Can you work these out from the model? Positions are in its coordinate system, mm. A direction names the side the tool comes from. Coordinates: 2 decimals unless noted, no trailing zeros. Write each loop counter-clockwise with the first axis right and the second up, starting at its lowest first coordinate (ties: lowest second). Pieces come first, ordered by that corner, then holes. Notation, with made-up numbers: M 59.25,13.25 L 88.25,13.25 A23 ccw 88.25,46.25 Z; hole C -33,3.25 d10. An arc over 180 degrees is marked long. Use one line per item in the form item = value. Start each with the question number.
```python
from build123d import *

# Parameters (mm, degrees)
SKETCH1_W           = 3
SKETCH1_H           = 7
BOSS_EXTRUDE1_DEPTH = 6
SKETCH5_W           = 70
SKETCH5_H           = 6
CUT_EXTRUDE2_DEPTH  = 2
SKETCH6_R           = 3
CUT_EXTRUDE3_DEPTH  = 10


with BuildPart() as part:
    # Sketch1 → Boss-Extrude1 (new body)
    # profile 1 of 3: a face of its own
    with BuildSketch(Plane.XY):
        with BuildLine():
            ThreePointArc((0.112083698, 404.617647059), (2.612083698, 407.117647059), (5.112083698, 404.617647059))
            Line((5.112083698, 404.617647059), (18.529411765, 404.617647059))
            Line((18.529411765, 404.617647059), (18.529411765, 419.117647059))
            ThreePointArc((18.529411765, 419.117647059), (17.064945671, 422.653180965), (13.529411765, 424.117647059))
            Line((13.529411765, 424.117647059), (-46.470588235, 424.117647059))
            ThreePointArc((-46.470588235, 424.117647059), (-50.006122141, 422.653180965), (-51.470588235, 419.117647059))
            Line((-51.470588235, 419.117647059), (-51.470588235, 404.617647059))
            Line((-51.470588235, 404.617647059), (-42.310598324, 404.617647059))
            ThreePointArc((-42.310598324, 404.617647059), (-39.810598324, 407.117647059), (-37.310598324, 404.617647059))
            Line((-37.310598324, 404.617647059), (0.112083698, 404.617647059))
        make_face()
    # profile 2 of 3: a face of its own
    with BuildSketch(Plane.XY):
        with BuildLine():
            Line((18.529411765, 404.617647059), (5.112083698, 404.617647059))
            ThreePointArc((5.112083698, 404.617647059), (2.612083698, 402.117647059), (0.112083698, 404.617647059))
            Line((0.112083698, 404.617647059), (-37.310598324, 404.617647059))
            ThreePointArc((-37.310598324, 404.617647059), (-39.810598324, 402.117647059), (-42.310598324, 404.617647059))
            Line((-42.310598324, 404.617647059), (-51.470588235, 404.617647059))
            Line((-51.470588235, 404.617647059), (-51.470588235, 373.617647059))
            Line((-51.470588235, 373.617647059), (-42.310598324, 373.617647059))
            ThreePointArc((-42.310598324, 373.617647059), (-39.810598324, 376.117647059), (-37.310598324, 373.617647059))
            Line((-37.310598324, 373.617647059), (0.112083698, 373.617647059))
            ThreePointArc((0.112083698, 373.617647059), (2.612083698, 376.117647059), (5.112083698, 373.617647059))
            Line((5.112083698, 373.617647059), (18.529411765, 373.617647059))
            Line((18.529411765, 373.617647059), (18.529411765, 404.617647059))
        make_face()
        with Locations((-46.970588235, 389.117647059)):
            Rectangle(SKETCH1_W, SKETCH1_H, mode=Mode.SUBTRACT)
        with Locations((14.029411765, 389.117647059)):
            Rectangle(SKETCH1_W, SKETCH1_H, mode=Mode.SUBTRACT)
    # profile 3 of 3: a face of its own
    with BuildSketch(Plane.XY):
        with BuildLine():
            Line((18.529411765, 359.117647059), (18.529411765, 373.617647059))
            Line((18.529411765, 373.617647059), (5.112083698, 373.617647059))
            ThreePointArc((5.112083698, 373.617647059), (2.612083698, 371.117647059), (0.112083698, 373.617647059))
            Line((0.112083698, 373.617647059), (-37.310598324, 373.617647059))
            ThreePointArc((-37.310598324, 373.617647059), (-39.810598324, 371.117647059), (-42.310598324, 373.617647059))
            Line((-42.310598324, 373.617647059), (-51.470588235, 373.617647059))
            Line((-51.470588235, 373.617647059), (-51.470588235, 359.117647059))
            ThreePointArc((-51.470588235, 359.117647059), (-50.006122141, 355.582113153), (-46.470588235, 354.117647059))
            Line((-46.470588235, 354.117647059), (13.529411765, 354.117647059))
            ThreePointArc((13.529411765, 354.117647059), (17.064945671, 355.582113153), (18.529411765, 359.117647059))
        make_face()
    extrude(amount=BOSS_EXTRUDE1_DEPTH)

    # Sketch5 → Cut-Extrude2 (cut)
    with BuildSketch(Plane.XY.offset(6)):
        with Locations((-16.470588235, 389.117647059)):
            Rectangle(SKETCH5_W, SKETCH5_H)
    extrude(amount=-CUT_EXTRUDE2_DEPTH, mode=Mode.SUBTRACT)

    # Sketch6 → Cut-Extrude3 (cut)
    with BuildSketch(Plane.XY.offset(4)):
        with Locations((-16.470588235, 389.117647059)):
            Circle(SKETCH6_R)
    extrude(amount=-CUT_EXTRUDE3_DEPTH, mode=Mode.SUBTRACT)


solid = part.part
```
1) Suppose I cut it at B-B on x = 4. Please give me the cut outline in (y, z).
2) Suppose I cut it at D-D on y = 372.5. Please give me the cut outline in (x, z).
3) Suppose I cut it at A-A on y = 387.5. Please give me the cut outline in (x, z).
4) Please list where these lines run through material, in increasing order: line 1 (Y direction, x = -40, z = 4.75); line 2 (Y direction, x = -26.5, z = 4.95); line 3 (Y direction, x = -39, z = 4.95).
5) Which directions (+Z, -Z, +X, -X, +Y, -Y) give clear straight access to the entire face, cutting with the end or side of a thin tool? Please do faces 1 (the face through (-47, 392.618, 3)), 2 (the face through (17.104, 422.614, 2.958)), 3 (the face through (-17, 386.118, 5)).
6) If we mould it in two halves opening along Y, with no side actions, what happens to faces 4 (the face through (17, 392.118, 5)), 5 (the face through (-2, 389, 4)), 6 (the face through (-17, 370, 6)), 7 (the face through (17.026, 355.543, 2.958))? For each: +Y half, -Y half, draft (parallel to the pull), parting line (faces both ways), or undercut.
7) Will these pins go through, and if not, where does the flat tip stop? pin 1 Ø4 at (x, y) = (2.61, 404.62) entering from -Z; pin 2 Ø5 at (x, y) = (-27, 389.5) entering from +Z; pin 3 Ø1 at (x, z) = (17, 5) entering from -Y; pin 4 Ø1.6 at (x, z) = (16.5, 5) entering from +Y.
8) Suppose I cut it at C-C on z = 2.1. Please give me the cut outline in (x, y), and give its area (3 significant figures).
Computed values:
q1.outline = M 354.12,0 L 371.54,0 L 371.54,6 L 354.12,6 Z; M 375.7,0 L 402.54,0 L 402.54,6 L 392.12,6 L 392.12,4 L 386.12,4 L 386.12,6 L 375.7,6 Z; M 406.7,0 L 424.12,0 L 424.12,6 L 406.7,6 Z
q2.outline = M -51.47,0 L -42.05,0 L -42.05,6 L -51.47,6 Z; M -37.57,0 L 0.38,0 L 0.38,6 L -37.57,6 Z; M 4.85,0 L 18.53,0 L 18.53,6 L 4.85,6 Z
q3.outline = M -51.47,0 L -48.47,0 L -48.47,4 L -51.47,4 Z; M -45.47,0 L -19,0 L -19,4 L -45.47,4 Z; M -13.94,0 L 12.53,0 L 12.53,4 L -13.94,4 Z; M 15.53,0 L 18.53,0 L 18.53,4 L 15.53,4 Z
q4.line_1 = 354.12 to 371.12, 376.11 to 386.12, 392.12 to 402.12, 407.11 to 424.12
q4.line_2 = 354.12 to 386.12, 392.12 to 424.12
q4.line_3 = 354.12 to 371.25, 375.98 to 386.12, 392.12 to 402.25, 406.98 to 424.12
q5.face_1 = +Z, -Z
q5.face_2 = +Z, -Z, +X, +Y
q5.face_3 = +Z, +X, -X
q6.face_4 = undercut
q6.face_5 = undercut
q6.face_6 = draft
q6.face_7 = -Y half
q7.pin_1 = through
q7.pin_2 = 4
q7.pin_3 = 355.1
q7.pin_4 = 423.62
q8.outline = M -51.47,359.12 A5 ccw -46.47,354.12 L 13.53,354.12 A5 ccw 18.53,359.12 L 18.53,419.12 A5 ccw 13.53,424.12 L -46.47,424.12 A5 ccw -51.47,419.12 Z; hole M -48.47,385.62 L -45.47,385.62 L -45.47,392.62 L -48.47,392.62 Z; hole C -39.81,373.62 d5; hole C -39.81,404.62 d5; hole C -16.47,389.12 d6; hole C 2.61,373.62 d5; hole C 2.61,404.62 d5; hole M 12.53,385.62 L 15.53,385.62 L 15.53,392.62 L 12.53,392.62 Z
q8.area = 4,730 mm²
